Part model, mm, in its own coordinate system. A direction names the side the tool comes from. Give positions to 0.01 mm unless a question says otherwise; leave off trailing zeros. Order: outer loops, then holes, each group sorted by start corner. A loop starts at its lowest first (then second) coordinate and runs counter-clockwise, first axis right, second up. Notation, with made-up numbers: (-24, 85) - (15, 85) arc R34 ccw to (15, 124) - close; hole circle Ø8 at (5, 31.5). An arc over 180 degrees is marked (long way). Use a Markdown table: item, result. Add a question column.
from build123d import *

# Parameters (mm, degrees)
EXTRUDE_THIN1_START       = -250
EXTRUDE_THIN1_OUTLINE_W   = 1000
EXTRUDE_THIN1_OUTLINE_H   = 500
EXTRUDE_THIN1_OUTLINE_W_2 = 996
EXTRUDE_THIN1_OUTLINE_H_2 = 496
EXTRUDE_THIN1_DEPTH       = 750
EXTRUDE_THIN2_START       = -498
SKETCH2_W                 = 500
SKETCH2_H                 = 1000
SKETCH2_W_2               = 496
SKETCH2_H_2               = 996
EXTRUDE_THIN2_DEPTH       = 748
CUT_EXTRUDE1_REACH        = 1032.776
SKETCH3_W                 = 496
SKETCH3_H                 = 996
CUT_EXTRUDE2_REACH        = 1032.776
SKETCH4_W                 = 996
SKETCH4_H                 = 496


# Read off the part's stored shape, not the designer's step: Extrude-Thin1
with BuildPart() as part:
    # Extrude-Thin1 outline → Extrude-Thin1 (new body)
    with BuildSketch(Plane(origin=(0, 0, 0), x_dir=(0, 0, -1), z_dir=(1, 0, 0)).offset(EXTRUDE_THIN1_START)):
        Rectangle(EXTRUDE_THIN1_OUTLINE_W, EXTRUDE_THIN1_OUTLINE_H)
        Rectangle(EXTRUDE_THIN1_OUTLINE_W_2, EXTRUDE_THIN1_OUTLINE_H_2, mode=Mode.SUBTRACT)
    extrude(amount=EXTRUDE_THIN1_DEPTH)

    # Sketch2 → Extrude-Thin2 (add)
    with BuildSketch(Plane.XZ.offset(250).offset(EXTRUDE_THIN2_START)):
        Rectangle(SKETCH2_W, SKETCH2_H)
        Rectangle(SKETCH2_W_2, SKETCH2_H_2, mode=Mode.SUBTRACT)
    extrude(amount=EXTRUDE_THIN2_DEPTH)

    # Sketch3 → Cut-Extrude1 (cut, up to next)
    with BuildSketch(Plane.XZ.offset(500), mode=Mode.PRIVATE) as cut_extrude1_sk1:
        Rectangle(SKETCH3_W, SKETCH3_H)
    cut_extrude1_tool1 = extrude(cut_extrude1_sk1.sketch, amount=-CUT_EXTRUDE1_REACH, mode=Mode.PRIVATE) & part.part
    add(cut_extrude1_tool1.solids().sort_by_distance((0, -500, 0))[0], mode=Mode.SUBTRACT)

    # Sketch4 → Cut-Extrude2 (cut, up to next)
    with BuildSketch(Plane(origin=(500, 0, 0), x_dir=(0, 0, -1), z_dir=(1, 0, 0)), mode=Mode.PRIVATE) as cut_extrude2_sk1:
        Rectangle(SKETCH4_W, SKETCH4_H)
    cut_extrude2_tool1 = extrude(cut_extrude2_sk1.sketch, amount=-CUT_EXTRUDE2_REACH, mode=Mode.PRIVATE) & part.part
    add(cut_extrude2_tool1.solids().sort_by_distance((500, 0, 0))[0], mode=Mode.SUBTRACT)


solid = part.part
1. Mould opens along Z. For faces 1 (the face through (373, -250, 7)), 2 (the face through (120, -120, -500)), 3 (the face through (121, -121, -498)), 4 (the face through (120, -120, 500)) say: released by +Z, released by -Z, zero draft, split by the parting line, or undercut.
2. Cut at A-A (z = -55). Write the cut outline in (x, y).
3. Pin check, flat tips, straight feed: P1, Ø5, axis at x = -146, z = 104, coming from the -Y side; P2, Ø6, axis at y = 31, z = -310.5, coming from the +X side; P3, Ø6, axis at x = 404.5, z = -129, coming from the -Y side. Stop position of each tip, or through.
4. Cut at D-D (y = -230). Write the cut outline in (x, z).
5. Cut at B-B (x = 398.5). Write the cut outline in (y, z), plus the area to 3 significant figures.
6. Tool access for faces 5 (the face through (121, 248, 7)), 6 (the face through (121, -121, 498)), 7 (the face through (250, -373, -7)), 8 (the face through (120, 250, 7)), 9 (the face through (248, -372, -7)): list every direction of +Z, -Z, +X, -X, +Y, -Y with a clear straight run to the whole face (end or side of a thin tool).
7. Drill centre lines: probe 1 along Z at (x, y) = (-156.5, 193); probe 2 along Y at (x, z) = (334, -90.5). Where is each one in solid material? Low to high. Write a range as [from, to].
Responses:
| question | item | result |
|---|---|---|
| 1 | face 1 | zero draft |
| 1 | face 2 | released by -Z |
| 1 | face 3 | undercut |
| 1 | face 4 | released by +Z |
| 2 | outline | (-250, -500) - (-248, -500) - (-248, 248) - (500, 248) - (500, 250) - (-250, 250) - close; (248, -500) - (250, -500) - (250, -250) - (500, -250) - (500, -248) - (248, -248) - close |
| 3 | P1 | stops at y = 248 |
| 3 | P2 | stops at x = -248 |
| 3 | P3 | stops at y = -250 |
| 4 | outline | (-250, -500) - (500, -500) - (500, -498) - (-248, -498) - (-248, 498) - (500, 498) - (500, 500) - (-250, 500) - close |
| 5 | outline | (-250, -500) - (250, -500) - (250, 500) - (-250, 500) - close; hole (-248, -498) - (248, -498) - (248, 498) - (-248, 498) - close |
| 5 | area | 5,980 mm² |
| 6 | face 5 | +X |
| 6 | face 6 | none |
| 6 | face 7 | +Z, -Z, +X, -Y |
| 6 | face 8 | +Z, -Z, +X, -X, +Y |
| 6 | face 9 | -Y |
| 7 | probe 1 | z = [-500, -498], [498, 500] |
| 7 | probe 2 | y = [-250, -248], [248, 250] |
